Design review of the part built by this model. Coordinates are the model's own, in mm. Face numbers are marked on the shaded views. Coordinates: 2 decimals unless noted, no trailing zeros. Write each loop counter-clockwise with the first axis right and the second up, starting at its lowest first coordinate (ties: lowest second). Pieces come first, ordered by that corner, then holes. Notation, with made-up numbers: M 25.5,17 L 33.5,17 A21 cw 33.5,35 Z; hole C 8.25,27 d8. An arc over 180 degrees is marked long. Return JSON: item names as keys, results as strings. Group by question number.
Autodesk Inventor part; units mm, degrees
ref_plane "YZ Plane" through (0, 0, 0) normal (1, 0, 0) x (0, 1, 0)
ref_plane "XZ Plane" through (0, 0, 0) normal (0, 1, 0) x (-1, 0, 0)
ref_plane "XY Plane" through (0, 0, 0) normal (0, 0, 1) x (1, 0, 0)
sketch "Sketch1" plane through (0, 0, 0) normal (0, 1, 0) x (-1, 0, 0)
  line L0 (66.5, 134) -> (-66.5, 134)
  line L1 (-66.5, 134) -> (-66.5, -134)
  line L2 (-66.5, -134) -> (66.5, -134)
  line L3 (66.5, -134) -> (66.5, 134)
  point P0 (0, 0)
  dimension "d0" = 133
  dimension "d1" = 268
  dimension "d2" = 66.5
  dimension "d3" = 134
extrude "Extrusion1" add sketch "Sketch1" along normal blind 20.3
shell "Shell1" thickness 3 removed faces 1 at (-22.1667, 0, -44.6667)
sketch "Sketch2" plane through (0, 20.3, 0) normal (0, 1, 0) x (1, 0, 0)
  line L0 (-53, 120.5) -> (53, 120.5)
  line L1 (53, 120.5) -> (53, -120.5)
  line L2 (53, -120.5) -> (-53, -120.5)
  line L3 (-53, -120.5) -> (-53, 120.5)
  line L4 (-66.5, 134) -> (-66.5, -134)
  line L5 (-66.5, -134) -> (66.5, -134)
  line L6 (66.5, -134) -> (66.5, 134)
  line L7 (66.5, 134) -> (-66.5, 134)
  point P0 (0, 0)
  dimension "d7" = 13.5
  dimension "d8" = 13.5
  dimension "d9" = 13.5
  dimension "d10" = 13.5
extrude "Extrusion2" cut sketch "Sketch2" against normal through all contours L0 L1 L2 L3
sketch "Sketch3" plane through (-63.5, 17.3, 131) normal (0, -1, 0) x (1, 0, 0)
  arc A0 (117, 0) -> (127, -10) centre (127, 0) ccw
  line L0 (127, 0) -> (127, -262)
  line L1 (0, 0) -> (127, 0)
  line L2 (127, -262) -> (0, -262)
  arc A1 (127, -252) -> (117, -262) centre (127, -262) ccw
  line L3 (0, -262) -> (0, 0)
  arc A2 (0, -10) -> (10, 0) centre (0, 0) ccw
  arc A3 (10, -262) -> (0, -252) centre (0, -262) ccw
  arc A4 (127, -123.5) -> (127, -138.5) centre (127, -131) ccw
  arc A5 (0, -138.5) -> (0, -123.5) centre (0, -131) ccw
  line L4 (127, 0) -> (124.6095, 0)
  line L5 (127, 0) -> (124.5, 0)
  line L6 (124.5, 0) -> (124.5, -262)
  line L7 (124.5, -262) -> (127, -262)
  line L8 (127, -262) -> (127, 0)
  line L9 (0, 0) -> (2.5, 0)
  line L10 (2.5, 0) -> (2.5, -262)
  line L11 (2.5, -262) -> (0, -262)
  line L12 (0, -262) -> (0, 0)
  line L13 (0, -262) -> (0, 0)
  line L14 (0, -262) -> (127, -262)
  line L15 (127, -262) -> (127, -259.5)
  line L16 (127, -259.5) -> (0, -259.5)
  line L17 (0, -259.5) -> (0, -262)
  line L18 (0, 0) -> (127, 0)
  line L19 (127, 0) -> (127, -2.5)
  line L20 (127, -2.5) -> (0, -2.5)
  line L21 (0, -2.5) -> (0, 0)
  point P0 (63.5, -131)
  point P1 (9.6825, -259.5)
  point P2 (2.5, -252.3175)
  point P3 (2.5, -138.0711)
  point P4 (2.5, -123.9289)
  point P5 (2.5, -9.6825)
  point P6 (9.6825, -2.5)
  point P7 (117.3175, -2.5)
  point P8 (124.5, -9.6825)
  point P9 (124.5, -123.9289)
  point P10 (124.5, -138.0711)
  point P11 (124.5, -252.3175)
  point P12 (117.3175, -259.5)
  dimension "d13" = 20
  dimension "d14" = 0
  dimension "d15" = 0
  dimension "d16" = 20
  dimension "d17" = 20
  dimension "d18" = 20
  dimension "d19" = 15
  dimension "d20" = 15
  dimension "d21" = 0
  dimension "d22" = 0
  dimension "d24" = 0
  dimension "d25" = 0
  dimension "d28" = 2.5
  dimension "d29" = 0
  dimension "d30" = 0
  dimension "d31" = 0
  dimension "d32" = 2.5
  dimension "d33" = 0
  dimension "d34" = 2.5
  dimension "d35" = 0
  dimension "d36" = 2.5
  dimension "d37" = 0
extrude "Extrusion3" add sketch "Sketch3" along normal blind 21.3 contours L1 L6 L20 A0 | A0 L20 A2 L1 | L20 L6 A0 | A2 L20 L10 L1 | L1 L0 L20 L6 | L6 L20 L0 A0 | A0 L0 A4 L6 | A2 L10 L20 | L10 L20 L3 L1 | L6 A4 | A4 L0 L6 | L10 A5 L3 A2 | A2 L3 L20 L10 | A4 L0 A1 L6 | L10 A5 L3 | A5 L10 | L6 L16 A1 | A1 L0 L16 L6 | L10 A3 L3 A5 | L16 L6 L2 A1 | A1 L2 A3 L16 | L16 L0 L2 L6 | L10 L16 L3 A3 | A3 L16 L10 | A3 L2 L10 L16 | L10 L2 L3 L16
fillet "Fillet2" radius 4 4 edges at (-66.5, 10.15, -134) (-66.5, 10.15, 134) (66.5, 10.15, 134) (66.5, 10.15, -134)
fillet "Fillet3" radius 1 4 edges at (53, 18.8, 120.5) (53, 18.8, -120.5) (-53, 18.8, -120.5) (-53, 18.8, 120.5)
chamfer "Chamfer1" distance 2 angle 45 8 edges at (0, 20.3, 134) (65.3284, 20.3, 132.8284) (66.5, 20.3, 0) (65.3284, 20.3, -132.8284) (0, 20.3, -134) (-65.3284, 20.3, -132.8284) (-66.5, 20.3, 0) (-65.3284, 20.3, 132.8284)
sketch "Sketch4" plane through (-63.5, -4, 131) normal (0, -1, 0) x (1, 0, 0)
  circle A0 centre (123.75, -258.75) radius 1.75
  circle A1 centre (3.25, -258.75) radius 1.75
  circle A2 centre (3.25, -3.25) radius 1.75
  circle A3 centre (123.75, -3.25) radius 1.75
  circle A4 centre (123.75, -131) radius 1.75
  circle A5 centre (3.25, -131) radius 1.75
  point P0 (63.5, -131)
hole "Hole1" at (-60.25, -4, 127.75) at (60.25, -4, 127.75) at (60.25, -4, 0) at (60.25, -4, -127.75) at (-60.25, -4, -127.75) at (-60.25, -4, 0) direction (0, 1, 0) diameter 2.6 depth 6 tip angle 118
properties part number "Cover"
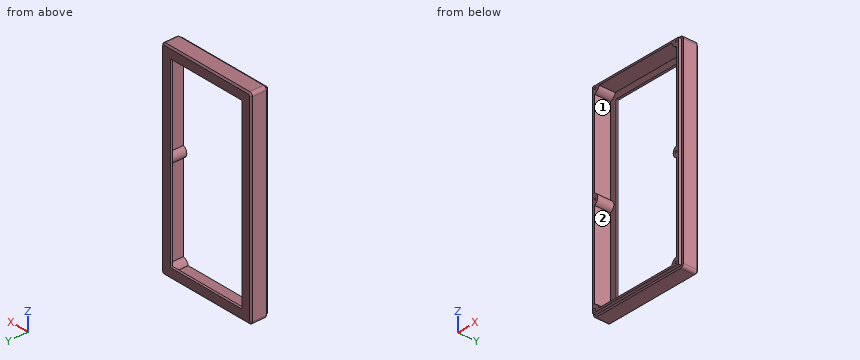
Item 1: Add section A-A (z = 87.5). Write out the cut boundary in (x, y).
Item 2: Add section C-C (y = 7.75). Write out the cut boundary in (x, z), plus the area to 3 significant figures.
Item 3: For pin 1 (2 mm diameter, centred on x = -60.25, z = 0, fed in from -Y); pin 2 (1.2 mm diameter, centred on y = -3, z = 0, fed in from +X); pin 3 (1.5 mm diameter, centred on x = -12, y = -1, fed in from +Z), all flat-tipped, find the tip position at first contact; note any pin that passes through.
Item 4: Add section B-B (x = -22). Write out the cut boundary in (y, z).
Item 5: For line 1 (Z direction, x = 50, y = 17.5); line 2 (Z direction, x = 34.5, y = 4); line 3 (X direction, y = 0.05, z = 127.75), list the stretches that pass through material, from the lowest coordinate up.
Item 6: The part is to be moulded in two halves that separate along X. For the marked faces 1 and 2, say which applies: pulls with the +X half, pulls with the -X half, needs draft (parallel to the pull), parting line crosses it, or undercut.
Geometry check:
{
 "1": {"outline": "M -66.5,0 L -63.5,0 L -63.5,-4 L -61,-4 L -61,17.3 L -53,17.3 L -53,20.3 L -64.5,20.3 L -66.5,18.3 Z; M 53,17.3 L 61,17.3 L 61,-4 L 63.5,-4 L 63.5,0 L 66.5,0 L 66.5,18.3 L 64.5,20.3 L 53,20.3 Z"},
 "2": {"outline": "M -66.5,-130 A4 ccw -62.5,-134 L 62.5,-134 A4 ccw 66.5,-130 L 66.5,130 A4 ccw 62.5,134 L -62.5,134 A4 ccw -66.5,130 Z; hole M -61,-121.32 A10 cw -53.82,-128.5 L 53.82,-128.5 A10 cw 61,-121.32 L 61,-7.07 A7.5 cw 61,7.07 L 61,121.32 A10 cw 53.82,128.5 L -53.82,128.5 A10 cw -61,121.32 L -61,7.07 A7.5 cw -61,-7.07 Z", "area": "4,520 mm^2"},
 "3": {"pin 1": "y = 2.18", "pin 2": "x = 63.5", "pin 3": "z = 131"},
 "4": {"outline": "M -4,-131 L 0,-131 L 0,-134 L 18.3,-134 L 20.3,-132 L 20.3,-120.5 L 17.3,-120.5 L 17.3,-128.5 L -4,-128.5 Z; M -4,128.5 L 17.3,128.5 L 17.3,120.5 L 20.3,120.5 L 20.3,132 L 18.3,134 L 0,134 L 0,131 L -4,131 Z"},
 "5": {"line 1": "-134 to -120.5, 120.5 to 134", "line 2": "-134 to -128.5, 128.5 to 134", "line 3": "-66.5 to -61.55, -58.95 to -54.04, 54.04 to 58.95, 61.55 to 66.5"},
 "6": {"face 1": "undercut", "face 2": "undercut"}
}
